Verification items for this drawing (mm, ordinates from the low corner). Give positions to 0.01 mm unless a question says otherwise; leave off trailing zeros. Loops run counter-clockwise (first coordinate to the right, second up) from the corner with the lowest first, then second, coordinate; pieces in that order, holes last. Notation, with made-up numbers: (73.5, 81.25) -> (86.5, 81.25) arc R9 ccw to (86.5, 85.25) -> close; hole circle Ø5 at (61, -33.75). An arc over 180 degrees is marked (long way). Write item = value, one per line.
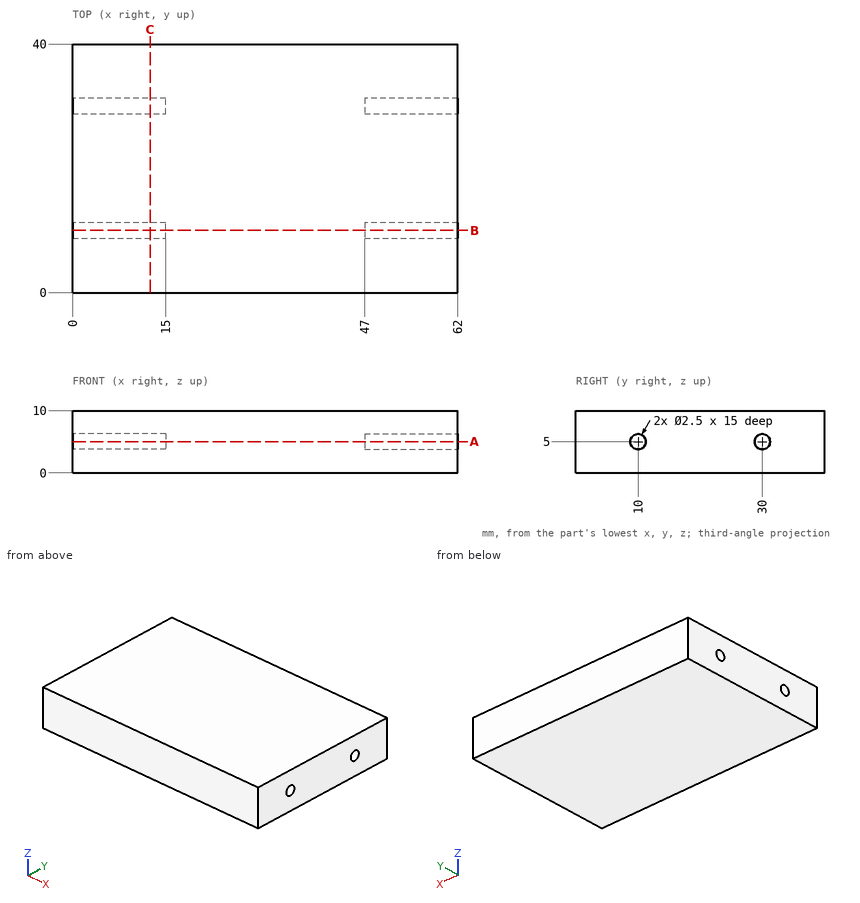
Item 1: Thickness scan on L1, parallel to Z at x = 54, y = 10. Record the ranges inside material, lowest first. Write a range as [from, to].
Answer:
L1 = [0, 3.75], [6.25, 10]
Item 2: Section check A-A, the plane z = 5. Record the cut outline in (x, y).
Answer:
outline = (0, 0) -> (62, 0) -> (62, 8.75) -> (47, 8.75) -> (47, 11.25) -> (62, 11.25) -> (62, 28.75) -> (47, 28.75) -> (47, 31.25) -> (62, 31.25) -> (62, 40) -> (0, 40) -> (0, 31.25) -> (15, 31.25) -> (15, 28.75) -> (0, 28.75) -> (0, 11.25) -> (15, 11.25) -> (15, 8.75) -> (0, 8.75) -> close
Item 3: Gauge pin test, flat ends, axial feed: pin 1 (0.8 mm diameter, centred on y = 10, z = 5, fed in from -X); pin 2 (0.8 mm diameter, centred on y = 29.5, z = 4.5, fed in from +X). Record the tip position at first contact, or that the pin passes through.
Answer:
pin_1 = 15
pin_2 = 47
Item 4: Section check B-B, the plane y = 10. Record the cut outline in (x, z).
Answer:
outline = (0, 0) -> (62, 0) -> (62, 3.75) -> (47, 3.75) -> (47, 6.25) -> (62, 6.25) -> (62, 10) -> (0, 10) -> (0, 6.25) -> (15, 6.25) -> (15, 3.75) -> (0, 3.75) -> close
Item 5: Section check C-C, the plane x = 12.5. Record the cut outline in (y, z), plus the area to 3 significant figures.
Answer:
outline = (0, 0) -> (40, 0) -> (40, 10) -> (0, 10) -> close; hole circle Ø2.5 at (10, 5); hole circle Ø2.5 at (30, 5)
area = 390 mm^2
